Input: part model. Units: mm. Frame: model coordinates. Give positions to 0.01 mm unless a question says otherwise; leave off trailing zeros. Write each loop counter-clockwise with the first axis right and the second up, starting at its lowest first coordinate (ties: lowest second). Pieces come first, ordered by that corner, then holes. Notation, with made-up numbers: (26, 32) -> (60, 32) arc R15 ccw to (60, 46) -> close; hole circle Ø9 at (43, -18.75). An arc over 180 degrees is marked (long way). Answer as a JSON object with one key per item and string values. Group by question number.
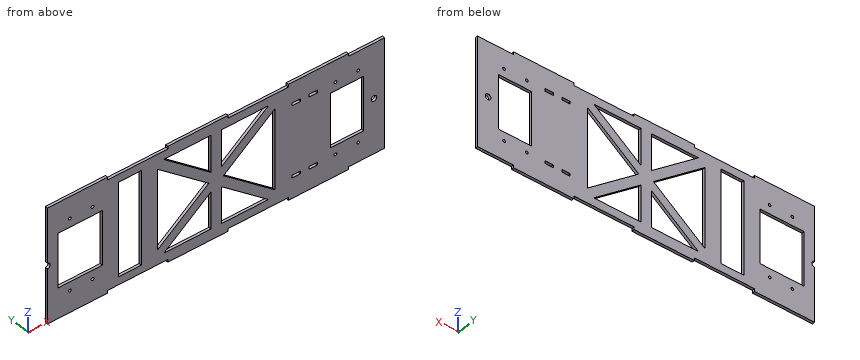
from build123d import *

# Parameters (mm, degrees)
F0_R     = 1.64084
F0_W     = 10
F0_H     = 3.175
F0_R_2   = 3.302
F0_W_2   = 52.4243835688
F0_H_2   = 64.2
F0_W_3   = 27.0990398764
F0_H_3   = 111.2592631512
F0_W_4   = 39.0626990616
F1_DEPTH = 3.175


with BuildPart() as f1:
    # F0 (on Front) → F1 (new body)
    with BuildSketch(Plane.XZ):
        with BuildLine():
            Line((79.2994276966, -50.2024036679), (122.1565705538, -50.2024036679))
            Line((122.1565705538, -50.2024036679), (122.1565705538, 79.7975963321))
            Line((122.1565705538, 79.7975963321), (79.2994276966, 79.7975963321))
            Line((79.2994276966, 79.7975963321), (79.2994276966, 82.9725963321))
            Line((79.2994276966, 82.9725963321), (7.870856268, 82.9725963321))
            Line((7.870856268, 82.9725963321), (7.870856268, 79.7975963321))
            Line((7.870856268, 79.7975963321), (-63.5577151605, 79.7975963321))
            Line((-63.5577151605, 79.7975963321), (-63.5577151605, 82.9725963321))
            Line((-63.5577151605, 82.9725963321), (-134.9862865891, 82.9725963321))
            Line((-134.9862865891, 82.9725963321), (-134.9862865891, 79.7975963321))
            Line((-134.9862865891, 79.7975963321), (-206.4148580177, 79.7975963321))
            Line((-206.4148580177, 79.7975963321), (-206.4148580177, 82.9725963321))
            Line((-206.4148580177, 82.9725963321), (-277.8434294462, 82.9725963321))
            Line((-277.8434294462, 82.9725963321), (-277.8434294462, 79.7975963321))
            Line((-277.8434294462, 79.7975963321), (-277.8434294462, 18.0995963321))
            ThreePointArc((-277.8434294462, 18.0995963321), (-275.5085628548, 17.1324629236), (-274.5414294462, 14.7975963321))
            ThreePointArc((-274.5414294462, 14.7975963321), (-275.5085628548, 12.4627297406), (-277.8434294462, 11.4955963321))
            Line((-277.8434294462, 11.4955963321), (-277.8434294462, -50.2024036679))
            Line((-277.8434294462, -50.2024036679), (-277.8434294462, -53.3774036679))
            Line((-277.8434294462, -53.3774036679), (-206.4148580177, -53.3774036679))
            Line((-206.4148580177, -53.3774036679), (-206.4148580177, -50.2024036679))
            Line((-206.4148580177, -50.2024036679), (-134.9862865891, -50.2024036679))
            Line((-134.9862865891, -50.2024036679), (-134.9862865891, -53.3774036679))
            Line((-134.9862865891, -53.3774036679), (-63.5577151605, -53.3774036679))
            Line((-63.5577151605, -53.3774036679), (-63.5577151605, -50.2024036679))
            Line((-63.5577151605, -50.2024036679), (7.870856268, -50.2024036679))
            Line((7.870856268, -50.2024036679), (7.870856268, -53.3774036679))
            Line((7.870856268, -53.3774036679), (79.2994276966, -53.3774036679))
            Line((79.2994276966, -53.3774036679), (79.2994276966, -50.2024036679))
        make_face()
        with Locations((-251.3181294462, -27.6524106679)):
            Circle(F0_R, mode=Mode.SUBTRACT)
        with Locations((-224.3687294462, -27.6524106679)):
            Circle(F0_R, mode=Mode.SUBTRACT)
        with Locations((17.1565705538, -27.6524036679)):
            Rectangle(F0_W, F0_H, mode=Mode.SUBTRACT)
        with Locations((37.1565705538, -27.6524036679)):
            Rectangle(F0_W, F0_H, mode=Mode.SUBTRACT)
        with Locations((63.6818705538, -27.6524106672)):
            Circle(F0_R, mode=Mode.SUBTRACT)
        with Locations((90.6312705538, -27.6524106672)):
            Circle(F0_R, mode=Mode.SUBTRACT)
        Polygon((-8.1668528914, -32.7346504676), (-8.1668528914, -40.3546504676), (-15.7868528914, -40.3546504676), (-71.6971936822, -40.3546504676), (-83.9896652103, -40.3546504676), (-139.900006001, -40.3546504676), (-147.520006001, -40.3546504676), (-147.520006001, -32.7346504676), (-147.520006001, 62.3298431318), (-147.520006001, 69.9498431318), (-139.900006001, 69.9498431318), (-83.9896652103, 69.9498431318), (-71.6971936822, 69.9498431318), (-15.7868528915, 69.9498431318), (-8.1668528914, 69.9498431318), (-8.1668528914, 62.3298431318), align=None, mode=Mode.SUBTRACT)
        with Locations((109.4565705538, 14.7975963321)):
            Circle(F0_R_2, mode=Mode.SUBTRACT)
        with Locations((-238.9312376618, 14.7975963321)):
            Rectangle(F0_W_2, F0_H_2, mode=Mode.SUBTRACT)
        with Locations((-180.1195259392, 14.7975963321)):
            Rectangle(F0_W_3, F0_H_3, mode=Mode.SUBTRACT)
        with Locations((-251.3181294462, 57.2475963321)):
            Circle(F0_R, mode=Mode.SUBTRACT)
        with Locations((-224.3687294462, 57.2475963321)):
            Circle(F0_R, mode=Mode.SUBTRACT)
        with Locations((77.5555704206, 15.0792245534)):
            Rectangle(F0_W_4, F0_H_2, mode=Mode.SUBTRACT)
        with Locations((17.1565705538, 57.2475963321)):
            Rectangle(F0_W, F0_H, mode=Mode.SUBTRACT)
        with Locations((37.1565705538, 57.2475963321)):
            Rectangle(F0_W, F0_H, mode=Mode.SUBTRACT)
        with Locations((63.6818705538, 57.2475963321)):
            Circle(F0_R, mode=Mode.SUBTRACT)
        with Locations((90.6312705538, 57.2475963321)):
            Circle(F0_R, mode=Mode.SUBTRACT)
        Polygon((-147.520006001, 62.3298431318), (-86.5412493668, 14.7975963321), (-83.9896652103, 16.7865271426), (-83.9896652103, 26.3683687987), (-139.900006001, 69.9498431318), (-147.520006001, 69.9498431318), align=None)
        Polygon((-69.1456095257, 14.7975963321), (-8.1668528915, 62.3298431318), (-8.1668528914, 69.9498431318), (-15.7868528915, 69.9498431318), (-71.6971936822, 26.3683687987), (-71.6971936822, 16.7865271426), align=None)
        Polygon((-15.7868528914, -40.3546504676), (-8.1668528914, -40.3546504676), (-8.1668528914, -32.7346504676), (-69.1456095257, 14.7975963321), (-71.6971936822, 12.8086655216), (-71.6971936822, 3.2268238655), align=None)
        Polygon((-147.520006001, -40.3546504676), (-139.900006001, -40.3546504676), (-83.9896652103, 3.2268238655), (-83.9896652103, 12.8086655216), (-86.5412493668, 14.7975963321), (-147.520006001, -32.7346504676), align=None)
        Polygon((-83.9896652103, -40.3546504676), (-71.6971936822, -40.3546504676), (-71.6971936822, 3.2268238655), (-77.8434294462, 8.0177446936), (-83.9896652103, 3.2268238655), align=None)
        Polygon((-77.8434294462, 8.0177446936), (-71.6971936822, 3.2268238655), (-71.6971936822, 12.8086655216), align=None)
        Polygon((-83.9896652103, 3.2268238655), (-77.8434294462, 8.0177446936), (-83.9896652103, 12.8086655216), align=None)
        Polygon((-86.5412493668, 14.7975963321), (-83.9896652103, 12.8086655216), (-83.9896652103, 16.7865271426), align=None)
        Polygon((-83.9896652103, 12.8086655216), (-77.8434294462, 8.0177446936), (-71.6971936822, 12.8086655216), (-71.6971936822, 16.7865271426), (-77.8434294462, 21.5774479707), (-83.9896652103, 16.7865271426), align=None)
        Polygon((-77.8434294462, 21.5774479707), (-71.6971936822, 16.7865271426), (-71.6971936822, 26.3683687987), align=None)
        Polygon((-83.9896652103, 16.7865271426), (-77.8434294462, 21.5774479707), (-83.9896652103, 26.3683687987), align=None)
        Polygon((-83.9896652103, 26.3683687987), (-77.8434294462, 21.5774479707), (-71.6971936822, 26.3683687987), (-71.6971936822, 69.9498431318), (-83.9896652103, 69.9498431318), align=None)
        Polygon((-71.6971936822, 12.8086655216), (-69.1456095257, 14.7975963321), (-71.6971936822, 16.7865271426), align=None)
    extrude(amount=F1_DEPTH)


solid = f1.part
1. Contact query for flat-ended pins moving along their axis: pin 1 Ø1 at (y, z) = (-2, 81) entering from +X; pin 2 Ø3 at (x, z) = (-251.32, 57.25) entering from +Y (3 decimals); pin 3 Ø1.6 at (x, y) = (111, -1.5) entering from +Z. Output: stop coordinate, or through.
2. Section B-B (z = -6.5). State how many separate pieces and enclosed holes the cut face has, plus the area to 3 significant figures.
3. Section A-A (x = -188). Return the cut outline in (y, z) (3 decimals).
4. Line query: line 1 (Z direction, x = 19, y = -1.2); line 2 (Z direction, x = 72.5, y = -0.5); line 3 (X direction, y = -2.85, z = -34). Output: solid intervals per line, ascending.
Working result:
{
 "1": {"pin 1": "stops at x = 79.3", "pin 2": "passes through", "pin 3": "stops at z = 79.8"},
 "2": {"separate pieces": "8", "enclosed holes": "0", "area": "601 mm^2"},
 "3": {"outline": "(-3.175, -50.202) -> (0, -50.202) -> (0, -40.832) -> (-3.175, -40.832) -> close; (-3.175, 70.427) -> (0, 70.427) -> (0, 79.798) -> (-3.175, 79.798) -> close"},
 "4": {"line 1": "z = -53.38 to -29.24, -26.06 to 55.66, 58.84 to 82.97", "line 2": "z = -53.38 to -17.02, 47.18 to 82.97", "line 3": "x = -277.84 to -193.67, -166.57 to -131.75, -83.99 to -71.7, -23.94 to 122.16"}
}
